The model under review builds one solid part; all positions refer to its coordinate system, in mm. A direction names the side the tool comes from. Round coordinates to 2 decimals unless told otherwise and drop trailing zeros. Order: outer loops, then holes, each group sorted by start corner. A loop starts at its lowest first (then second) coordinate and runs counter-clockwise, first axis right, second up. Notation, with made-up numbers: (42, -0.5) -> (94, -0.5) arc R16 cw to (94, 18.5) -> close; hole circle Ø5 at (3.25, 76.25). An arc over 180 degrees is marked (long way). Return JSON: item names as keys, results as strings. Group by question number.
from build123d import *

# Parameters (mm, degrees)
SKETCH_R        = 11.3
SKETCH_R_2      = 1.6
SKETCH_R_3      = 3.2
PAD_DEPTH       = 15
SKETCH001_R     = 3.2
POCKET_DEPTH    = 4
SKETCH002_R     = 5.4
POCKET001_DEPTH = 4


with BuildPart() as part:
    # Sketch → Pad (new body)
    with BuildSketch(Plane.XY):
        Polygon((20, 30), (20, 50.15), (62.3, 50.15), (62.3, 30), (82.3, 30), (82.3, 0), (0, 0), (0, 30), align=None)
        with Locations((41.15, 29)):
            Circle(SKETCH_R, mode=Mode.SUBTRACT)
        with Locations((25.65, 44.5)):
            Circle(SKETCH_R_2, mode=Mode.SUBTRACT)
        with Locations((25.65, 13.5)):
            Circle(SKETCH_R_2, mode=Mode.SUBTRACT)
        with Locations((56.65, 44.5)):
            Circle(SKETCH_R_2, mode=Mode.SUBTRACT)
        with Locations((56.65, 13.5)):
            Circle(SKETCH_R_2, mode=Mode.SUBTRACT)
        with Locations((11.15, 10)):
            Circle(SKETCH_R_3, mode=Mode.SUBTRACT)
        with Locations((67.35, 10)):
            Circle(SKETCH_R_3, mode=Mode.SUBTRACT)
        with Locations((78.75, 10)):
            Circle(SKETCH_R_3, mode=Mode.SUBTRACT)
    extrude(amount=PAD_DEPTH)

    # Sketch001 (on Face18 of Pad) → Pocket (cut)
    with BuildSketch(Plane.XY.offset(15)):
        with Locations((25.65, 45.35)):
            Circle(SKETCH001_R)
        with Locations((56.65, 45.35)):
            Circle(SKETCH001_R)
        with Locations((56.65, 14.35)):
            Circle(SKETCH001_R)
        with Locations((25.65, 14.35)):
            Circle(SKETCH001_R)
    extrude(amount=-POCKET_DEPTH, mode=Mode.SUBTRACT)

    # Sketch002 (on Face4 of Pocket) → Pocket001 (cut)
    with BuildSketch(Plane(origin=(0, 0, 0), x_dir=(1, 0, 0), z_dir=(0, 0, -1))):
        with Locations((11.15, -10)):
            Circle(SKETCH002_R)
        with Locations((67.35, -10)):
            Circle(SKETCH002_R)
        with Locations((78.75, -10)):
            Circle(SKETCH002_R)
    extrude(amount=-POCKET001_DEPTH, mode=Mode.SUBTRACT)


solid = part.part
Item 1: Wall thickness on line 1 along Y through (x, z) = (25.65, 5.5); line 2 along Y through (x, z) = (25.65, 12.3); line 3 along Y through (x, z) = (11.5, 12.75): over which ranges is each line inside the solid? List them lowest first.
Item 2: Consider section B-B on y = 10. State the section outline as (x, z) points.
Item 3: The part is to be moulded in two halves that separate along X. For faces 1 (the face through (82.3, 15, 7)), 2 (the face through (42, 0, 7)), 3 (the face through (73.353, 9.827, 1.972)), say which applies: +X half, -X half, draft (parallel to the pull), parting line (faces both ways), or undercut.
Item 4: Consider section A-A on x = 67.35. State the section outline as (y, z) points.
Item 5: For faces 4 (the face through (62.3, 40, 7)), 5 (the face through (55.9, 15.1, 11)), 6 (the face through (10, 30, 7)), 7 (the face through (75, 10, 4)), list the 3-axis set-ups (+Z, -Z, +X, -X, +Y, -Y) from which the entire face can be reached by the end or side of a thin tool; tool diameter is ignored.
Item 6: Consider section C-C on z = 6.5. Give the number of separate pieces and of enclosed holes in the cut face, plus the area to 3 significant figures.
Item 7: Insertion check: pin 1 Ø1.5 at (y, z) = (35, 12.5) entering from +X; pin 2 Ø5 at (x, y) = (78.75, 10) entering from +Z; pin 3 Ø5 at (x, y) = (25.65, 14.35) entering from +Z; pin 4 Ø9.5 at (x, y) = (78.75, 10) entering from -Z. Each pin has a flat end and moves straight along its axis. Give the tip position at first contact, or say it passes through.
Item 8: Consider section D-D on x = 25.65. State the section outline as (y, z) points, plus the area to 3 significant figures.
Values:
{
 "1": {"line 1": "0 to 11.9, 15.1 to 42.9, 46.1 to 50.15", "line 2": "0 to 11.15, 17.55 to 42.15, 48.55 to 50.15", "line 3": "0 to 6.82, 13.18 to 30"},
 "2": {"outline": "(0, 0) -> (5.75, 0) -> (5.75, 4) -> (7.95, 4) -> (7.95, 15) -> (0, 15) -> close; (14.35, 4) -> (16.55, 4) -> (16.55, 0) -> (61.95, 0) -> (61.95, 4) -> (64.15, 4) -> (64.15, 15) -> (14.35, 15) -> close; (70.55, 4) -> (72.75, 4) -> (72.75, 0) -> (73.35, 0) -> (73.35, 4) -> (75.55, 4) -> (75.55, 15) -> (70.55, 15) -> close; (81.95, 4) -> (82.3, 4) -> (82.3, 15) -> (81.95, 15) -> close"},
 "3": {"face 1": "+X half", "face 2": "draft", "face 3": "undercut"},
 "4": {"outline": "(0, 0) -> (4.6, 0) -> (4.6, 4) -> (6.8, 4) -> (6.8, 15) -> (0, 15) -> close; (13.2, 4) -> (15.4, 4) -> (15.4, 0) -> (30, 0) -> (30, 15) -> (13.2, 15) -> close"},
 "5": {"face 4": "+Z, -Z, +X, +Y", "face 5": "+Z", "face 6": "+Z, -Z, -X, +Y", "face 7": "-Z"},
 "6": {"separate pieces": "1", "enclosed holes": "8", "area": "2,790 mm^2"},
 "7": {"pin 1": "x = 62.3", "pin 2": "through", "pin 3": "z = 11", "pin 4": "z = 4"},
 "8": {"outline": "(0, 0) -> (11.9, 0) -> (11.9, 11) -> (11.15, 11) -> (11.15, 15) -> (0, 15) -> close; (15.1, 0) -> (42.9, 0) -> (42.9, 11) -> (42.15, 11) -> (42.15, 15) -> (17.55, 15) -> (17.55, 11) -> (15.1, 11) -> close; (46.1, 0) -> (50.15, 0) -> (50.15, 15) -> (48.55, 15) -> (48.55, 11) -> (46.1, 11) -> close", "area": "631 mm^2"}
}
